Autodesk Inventor part; units mm, degrees
ref_plane "作業平面1" through (0, 0, 1.4) normal (0, 0, 1) x (1, 0, 0)
ref_plane "作業平面2" through (0, 0, 1) normal (0, 0, -1) x (-1, 0, 0)
ref_plane "作業平面3" through (0, 0, 1.5) normal (0, 0, -1) x (-1, 0, 0)
sketch "スケッチ1" plane through (0, 0, 0) normal (0, 0, 1) x (1, 0, 0)
  circle A0 centre (0, 0) radius 2
  circle A1 centre (0, 0) radius 2.5
  circle A2 centre (0, 0) radius 4
  circle A3 centre (0, 0) radius 3.5
  dimension "d0" = 4
  dimension "d1" = 5
  dimension "d2" = 8
  dimension "d3" = 7
extrude "押し出し1" add sketch "スケッチ1" along normal blind 2.4
sketch "スケッチ2" plane through (0, 0, 2.4) normal (0, 0, 1) x (1, 0, 0)
  point P0 (0, 0)
ref_plane "作業平面1" through (0, 0, 1.4) normal (0, 0, 1) x (1, 0, 0)
ref_plane "作業平面2" through (0, 0, 1) normal (0, 0, -1) x (-1, 0, 0)
ref_plane "作業平面3" through (0, 0, 1.5) normal (0, 0, -1) x (-1, 0, 0)
sketch "スケッチ3" plane through (0, 0, 1.5) normal (0, 0, -1) x (-1, 0, 0)
  circle A0 centre (0, 3) radius 0.5
  circle A1 centre (0, 0) radius 3.5
  circle A2 centre (0, 0) radius 2.5
  line L0 (0, 3.5) -> (0, 2.5)
revolve "回転1" add sketch "スケッチ3" angle 360 about axis through (0, 3.5, 1.5) along (0, -1, 0) picked at (0.1674, 3.0997) contours A0 L0
pattern_circular "円形状パターン1" count 8 over 360 about axis through (0, 0, -10) along (0, 0, 1) of "回転1"
sketch "スケッチ4" plane through (0, 0, 1) normal (0, 0, -1) x (-1, 0, 0)
  circle A0 centre (0, 0) radius 2.5
  circle A1 centre (0, 0) radius 3.5
extrude "押し出し2" add sketch "スケッチ4" along normal blind 0.5
sketch "スケッチ5" plane through (0, 0, 1.4) normal (0, 0, 1) x (1, 0, 0)
  circle A0 centre (0, 0) radius 2.5
  circle A1 centre (0, 0) radius 3.5
extrude "押し出し3" add sketch "スケッチ5" along normal blind 0.5
sketch "スケッチ6" plane through (0, 0, 0) normal (0, 0, -1) x (-1, 0, 0)
  circle A0 centre (0, 0) radius 2
  circle A1 centre (0, 0) radius 4.6
  circle A2 centre (0, 0) radius 2
  dimension "d17" = 9.2
extrude "押し出し4" add sketch "スケッチ6" along normal blind 0.6
sketch "スケッチ7" plane through (0, 0, 0) normal (0, 0, -1) x (-1, 0, 0)
  point P0 (0, 0)
properties part number "φ4φ8ベアリングa" material "鋼 AISI 1006 85 HR"
The listing builds one solid part. Answer for the finished solid, in the listing's coordinates (mm). A direction names the side the tool comes from. Coordinates: 2 decimals unless noted, no trailing zeros. Loops run counter-clockwise (first coordinate to the right, second up) from the corner with the lowest first, then second, coordinate; pieces in that order, holes last. Notation, with made-up numbers: M 21.25,-27 L 40.25,-27 A26 cw 40.25,7 Z; hole C -34,54 d11. An arc over 180 degrees is marked long. Answer as a JSON object with one key per item and string values. Group by question number.
Item 1: Determine the mould class of faces 1 (the face through (-1, -2, -0.6)), 2 (the face through (-0.867, 3.905, 1.183)), 3 (the face through (-2.3, -1.5, 1)) for opening direction Y: +Y half, -Y half, draft (parallel to the pull), parting line (faces both ways), or undercut.
Item 2: This flat-tipped pin is pushed along its axis until it touches: P1, Ø1.5, axis at x = 1, z = 0, coming from the -Y side. Where does it stop, or does it pass through?
Item 3: Consider L1, parallel to Y at x = 0, z = 2.1; L2, parallel to Z at x = 3.25, y = 0.5; L3, parallel to Y at x = -0.5, z = 0.45. Determine where each line is inside the solid, lowest interval first.
Item 4: Section A-A (x = -1) is taken. Give the number of separate pieces and of enclosed holes in the cut face, and give its area (3 significant figures).
Item 5: Which of the six approach directions +Z, -Z, +X, -X, +Y, -Y give full straight-line access (tool end or side, diameter ignored) to faces 4 (the face through (3.233, 1.341, 0.246)), 5 (the face through (-1, 2, 2.4)), 6 (the face through (3.233, 1.341, 2.146))?
Item 6: Section C-C (y = 3.75) is taken. Write down the section's boundary in (x, z).
Item 7: Section D-D (z = 1.6) is taken. Write down the section's boundary in (x, y), and give its area (3 significant figures).
Solved:
{
 "1": {"face 1": "draft", "face 2": "parting line", "face 3": "undercut"},
 "2": {"P1": "stops at y = -4.59"},
 "3": {"L1": "y = -4 to -3.5, -2.5 to -2, 2 to 2.5, 3.5 to 4", "L2": "z = -0.6 to 0, 0.5 to 1, 1.4 to 1.9", "L3": "y = -3.97 to -3.46, -2.45 to -1.94, 1.94 to 2.45, 3.46 to 3.97"},
 "4": {"separate pieces": "2", "enclosed holes": "4", "area": "10.6 mm2"},
 "5": {"face 4": "none", "face 5": "+Z, +X, -X, +Y, -Y", "face 6": "+Z"},
 "6": {"outline": "M -2.66,-0.6 L 2.66,-0.6 L 2.66,0 L 1.39,0 L 1.39,2.4 L -1.39,2.4 L -1.39,0 L -2.66,0 Z"},
 "7": {"outline": "C 0,0 d8; hole C 0,0 d4", "area": "37.7 mm2"}
}
